```python
from build123d import *

# Parameters (mm, degrees)
F0_R     = 3
F0_R_2   = 2.5
F1_DEPTH = 20
F2_R     = 7
F2_R_2   = 6
F3_DEPTH = 6.35
F4_R     = 6
F4_R_2   = 2.5
F5_DEPTH = 1
F7_DEPTH = 12.7


with BuildPart() as f1:
    # F0 (on Top) → F1 (new body)
    with BuildSketch(Plane.XY):
        Circle(F0_R)
        Circle(F0_R_2, mode=Mode.SUBTRACT)
    extrude(amount=F1_DEPTH)



with BuildPart() as f3:
    # F2 (on Top) → F3 (new body)
    with BuildSketch(Plane.XY):
        Circle(F2_R)
        Circle(F2_R_2, mode=Mode.SUBTRACT)
    extrude(amount=-F3_DEPTH)


with BuildPart() as f1_1:
    add(f1.part)

    add(f3.part)  # F5 merges F3
    # F4 (on Top) → F5 (join)
    with BuildSketch(Plane.XY):
        Circle(F4_R)
        Circle(F4_R_2, mode=Mode.SUBTRACT)
    extrude(amount=-F5_DEPTH)

    # F6 (on Front) → F7 (cut, symmetric)
    with BuildSketch(Plane.XZ):
        Polygon((3, 20), (-3, 20), (3, 14), align=None)
    extrude(amount=F7_DEPTH, both=True, mode=Mode.SUBTRACT)


solid = f1_1.part
```
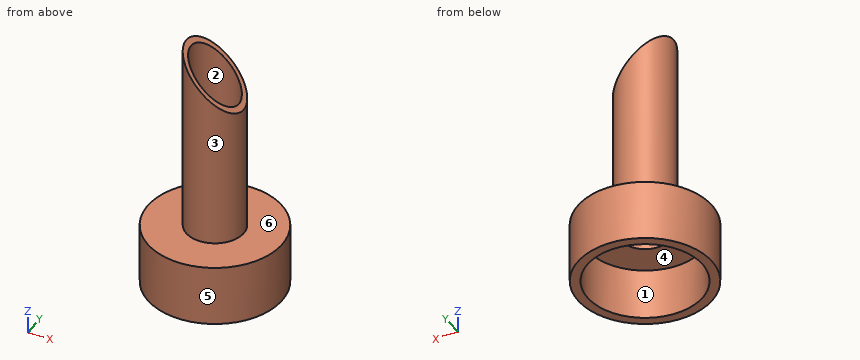
Geometry: final body of the model. Coordinates: model frame, mm. Face numbers are marked on the shaded views. A direction names the side the tool comes from. Round coordinates to 2 decimals unless told otherwise and drop trailing zeros. Write each loop counter-clockwise with the first axis right and the second up, starting at its lowest first coordinate (ties: lowest second). Pieces come first, ordered by that corner, then holes.
Item 1: Section query A-A (x = 0). Return loops of the section in (y, z), plus the area to 3 significant figures.
Item 2: Section query C-C (z = 4.25). Return loops of the section in (x, y), plus the area to 3 significant figures.
Item 3: Section query B-B (y = 0). Return loops of the section in (x, z), plus the area to 3 significant figures.
Item 4: Pin query (flat end, axial travel): P1, Ø2, axis at y = -0.5, z = -3.5, coming from the -X side; P2, Ø2, axis at x = -3.5, z = 5, coming from the +Y side; P3, Ø8, axis at y = 3.5, z = 9, coming from the -X side; P4, Ø5, axis at x = -4.5, z = 16.5, coming from the +Y side. Return the tip coordinate at first contact, or that it passes through.
Item 5: Set-up query: the marked faces 1, 2 and 3. Return all of +Z, -Z, +X, -X, +Y, -Y with unobstructed straight access to the full face (end or side cutting, diameter ignored); none if empty.
Item 6: Material intervals for L1, parallel to Y at x = 0, z = -2.45; L2, parallel to Y at x = 0, z = 13.75, sorted ascending.
Item 7: Mould query, pull axis X, two halves, no side actions, for the marked faces 4, 5 and 6. Classes: +X half, -X half, draft (parallel to the pull), parting line (faces both ways), or undercut.
Item 8: Section query D-D (y = -5.5). Return loops of the section in (x, z).
Completed:
1. outline: (-7, -6.35) - (-6, -6.35) - (-6, -1) - (-2.5, -1) - (-2.5, 17) - (-3, 17) - (-3, 0) - (-7, 0) - close; (2.5, -1) - (6, -1) - (6, -6.35) - (7, -6.35) - (7, 0) - (3, 0) - (3, 17) - (2.5, 17) - close
1. area: 36.7 mm2
2. outline: circle Ø6 at (0, 0); hole circle Ø5 at (0, 0)
2. area: 8.64 mm2
3. outline: (-7, -6.35) - (-6, -6.35) - (-6, -1) - (-2.5, -1) - (-2.5, 19.5) - (-3, 20) - (-3, 0) - (-7, 0) - close; (2.5, -1) - (6, -1) - (6, -6.35) - (7, -6.35) - (7, 0) - (3, 0) - (3, 14) - (2.5, 14.5) - close
3. area: 36.7 mm2
4. P1: stops at x = -7
4. P2: stops at y = 1.66
4. P3: stops at x = -3
4. P4: stops at y = 2.24
5. face 1: -Z
5. face 2: +Z, -Z
5. face 3: +Z
6. L1: y = -7 to -6, 6 to 7
6. L2: y = -3 to -2.5, 2.5 to 3
7. face 4: undercut
7. face 5: parting line
7. face 6: draft
8. outline: (-4.33, -6.35) - (-2.4, -6.35) - (-2.4, -1) - (2.4, -1) - (2.4, -6.35) - (4.33, -6.35) - (4.33, 0) - (-4.33, 0) - close
